Autodesk Inventor part; units mm, degrees
ref_plane "YZ Plane" through (0, 0, 0) normal (1, 0, 0) x (0, 1, 0)
ref_plane "XZ Plane" through (0, 0, 0) normal (0, 1, 0) x (-1, 0, 0)
ref_plane "XY Plane" through (0, 0, 0) normal (0, 0, 1) x (1, 0, 0)
sketch "Sketch1" plane through (0, 0, 0) normal (0, 0, 1) x (1, 0, 0)
  line L0 (17.5, -17.5) -> (0, -17.5)
  line L1 (-17.5, -17.5) -> (-17.5, 17.5)
  line L2 (-17.5, 17.5) -> (-7.5, 17.5) construction
  line L3 (17.5, 17.5) -> (17.5, 10)
  line L4 (17.5, -17.5) -> (-17.5, 17.5) construction
  line L5 (-17.5, -17.5) -> (17.5, 17.5) construction
  circle A0 centre (0, 0) radius 6.25
  line L6 (-17.5, -17.5) -> (-21.5, -17.5)
  line L7 (-21.5, -17.5) -> (-21.5, -7.5)
  line L8 (-21.5, -7.5) -> (-17.5, -7.5)
  line L9 (-17.5, -7.5) -> (-17.5, -17.5) construction
  line L10 (-17.5, 0) -> (-21.5, 0)
  line L11 (-21.5, 0) -> (-21.5, 10)
  line L12 (-21.5, 10) -> (-17.5, 10)
  line L13 (-17.5, 10) -> (-17.5, 0) construction
  line L14 (-17.5, 17.5) -> (-7.5, 17.5) construction
  line L15 (-7.5, 17.5) -> (-7.5, 21.5)
  line L16 (-7.5, 21.5) -> (-17.5, 21.5)
  line L17 (-17.5, 21.5) -> (-17.5, 17.5)
  line L18 (0, 17.5) -> (10, 17.5) construction
  line L19 (10, 17.5) -> (10, 21.5)
  line L20 (10, 21.5) -> (0, 21.5)
  line L21 (0, 21.5) -> (0, 17.5)
  line L22 (-17.5, 0) -> (17.5, 0) construction
  line L23 (0, -17.5) -> (0, 17.5) construction
  line L24 (-17.5, -17.5) -> (-7.5, -17.5)
  line L25 (-7.5, -17.5) -> (-7.5, -21.5)
  line L26 (-7.5, -21.5) -> (-17.5, -21.5)
  line L27 (-17.5, -21.5) -> (-17.5, -17.5)
  line L28 (0, -17.5) -> (10, -17.5) construction
  line L29 (10, -17.5) -> (10, -21.5)
  line L30 (10, -21.5) -> (0, -21.5)
  line L31 (0, -21.5) -> (0, -17.5)
  line L32 (17.5, -17.5) -> (21.5, -17.5)
  line L33 (21.5, -17.5) -> (21.5, -7.5)
  line L34 (21.5, -7.5) -> (17.5, -7.5)
  line L35 (17.5, -7.5) -> (17.5, -17.5) construction
  line L36 (17.5, 0) -> (21.5, 0)
  line L37 (21.5, 0) -> (21.5, 10)
  line L38 (21.5, 10) -> (17.5, 10)
  line L39 (17.5, 10) -> (17.5, 0) construction
  line L40 (-7.5, 17.5) -> (0, 17.5)
  line L41 (0, 17.5) -> (10, 17.5)
  line L42 (17.5, 10) -> (17.5, 0) construction
  line L43 (17.5, 0) -> (17.5, -7.5)
  line L44 (17.5, -7.5) -> (17.5, -17.5) construction
  line L45 (0, -17.5) -> (-17.5, -17.5)
  line L46 (10, 17.5) -> (17.5, 17.5)
  point P0 (0, 19.5)
  point P1 (-7.5, 19.5)
  point P2 (0, -19.5)
  point P3 (-7.5, -19.5)
  point P4 (-7.5, -17.5)
  point P5 (10, -17.5)
  dimension "d0" = 12.5
  dimension "d1" = 11.25
  dimension "d2" = 11.25
  dimension "d5" = 10
  dimension "d6" = 10
  dimension "d7" = 7.5
  dimension "d8" = 4
  dimension "d9" = 10
  dimension "d10" = 4
  dimension "d11" = 10
  dimension "d12" = 4
  dimension "d13" = 7.5
extrude "Extrusion1" add sketch "Sketch1" along normal blind 4
sketch "Sketch2" plane through (0, 0, 4) normal (0, 0, 1) x (1, 0, 0)
  line L0 (6.5, 17.5) -> (3.5, 17.5) construction
  line L1 (6.5, 21.5) -> (6.5, 17.5) construction
  line L2 (3.5, 21.5) -> (6.5, 21.5) construction
  line L3 (3.5, 21.5) -> (3.5, 17.5) construction
  line L4 (6.5, -21.5) -> (3.5, -21.5) construction
  line L5 (6.5, -17.5) -> (6.5, -21.5) construction
  line L6 (3.5, -17.5) -> (6.5, -17.5) construction
  line L7 (3.5, -17.5) -> (3.5, -21.5) construction
  line L8 (3.5, 17.5) -> (6.5, 21.5) construction
  line L9 (3.5, -17.5) -> (6.5, -21.5) construction
  circle A0 centre (5, 19.5) radius 1.5
  circle A1 centre (5, -19.5) radius 1.5
  point P0 (0, 0)
  dimension "d16" = 3
extrude "Extrusion2" cut sketch "Sketch2" against normal up to next
properties part number "FloorButtonHolder_Front_V1" material "MDF Medium Density Fiberboard"
Design review of the part built by this model. Coordinates are the model's own, in mm. A direction names the side the tool comes from. Give positions to 0.01 mm unless a question says otherwise; leave off trailing zeros. Order: outer loops, then holes, each group sorted by start corner. A loop starts at its lowest first (then second) coordinate and runs counter-clockwise, first axis right, second up. Notation, with made-up numbers: (50, 39) -> (64, 39) arc R18 cw to (64, 54) -> close; hole circle Ø1 at (-15.75, 47.5). An arc over 180 degrees is marked (long way). Write item = value, one per line. Start each with the question number.
(1) To check wall thickness, follow line 1 along Y through (x, z) = (19, 2.1); line 2 along Y through (x, z) = (5, 1.1); line 3 along X through (y, z) = (2, 0.65). State the ranges of each line that lie inside material, in increasing order.
(2) We need section C-C on x = -1.5. Write out the cut boundary in (y, z), plus the area to 3 significant figures.
(3) For faces 4 (the face through (-17.5, -4, 2)), 5 (the face through (-17.5, 16, 2)), 6 (the face through (-7.5, 19, 2)), 7 (the face through (10, 19, 2)), 8 (the face through (-17.5, -20, 2)), list the 3-axis set-ups (+Z, -Z, +X, -X, +Y, -Y) from which the entire face can be reached by the end or side of a thin tool; tool diameter is ignored.
(4) Mouldability with a two-part tool opening along X and no side actions: class faces 1 (the face through (-20, 10, 2)), 2 (the face through (0, 20, 2)), 3 (the face through (-21.5, 5, 2)) as +X half, -X half, draft (parallel to the pull), parting line (faces both ways), or undercut.
(5) We need section A-A on y = -19.5. Write out the cut boundary in (x, z), plus the area to 3 significant figures.
(6) We need section B-B on x = 5. Write out the cut boundary in (y, z), plus the area to 3 significant figures.
(7) For pin 1 (2 mm diameter, centred on x = 11.5, z = 3.5, fed in from -Y); pin 2 (1.2 mm diameter, centred on x = 19.5, z = 2, fed in from +Y); pin 3 (1.2 mm diameter, centred on x = 15.5, z = 1.5, fed in from +Y), all flat-tipped, find the tip position at first contact; note any pin that passes through.
(8) We need section D-D on y = -7. Write out the cut boundary in (x, z), plus the area to 3 significant figures.
Numbers:
q1.line_1 = -17.5 to -7.5, 0 to 10
q1.line_2 = -21.5 to -21, -18 to -3.75, 3.75 to 18, 21 to 21.5
q1.line_3 = -21.5 to -5.92, 5.92 to 21.5
q2.outline = (-17.5, 0) -> (-6.07, 0) -> (-6.07, 4) -> (-17.5, 4) -> close; (6.07, 0) -> (17.5, 0) -> (17.5, 4) -> (6.07, 4) -> close
q2.area = 91.5 mm^2
q3.face_4 = +Z, -Z, -X
q3.face_5 = +Z, -Z, -X, +Y
q3.face_6 = +Z, -Z, +Y
q3.face_7 = +Z, -Z, +X, +Y
q3.face_8 = +Z, -Z, -X, -Y
q4.face_1 = draft
q4.face_2 = undercut
q4.face_3 = -X half
q5.outline = (-17.5, 0) -> (-7.5, 0) -> (-7.5, 4) -> (-17.5, 4) -> close; (0, 0) -> (3.5, 0) -> (3.5, 4) -> (0, 4) -> close; (6.5, 0) -> (10, 0) -> (10, 4) -> (6.5, 4) -> close
q5.area = 68.0 mm^2
q6.outline = (-21.5, 0) -> (-21, 0) -> (-21, 4) -> (-21.5, 4) -> close; (-18, 0) -> (-3.75, 0) -> (-3.75, 4) -> (-18, 4) -> close; (3.75, 0) -> (18, 0) -> (18, 4) -> (3.75, 4) -> close; (21, 0) -> (21.5, 0) -> (21.5, 4) -> (21, 4) -> close
q6.area = 118 mm^2
q7.pin_1 = -17.5
q7.pin_2 = 10
q7.pin_3 = 17.5
q8.outline = (-17.5, 0) -> (17.5, 0) -> (17.5, 4) -> (-17.5, 4) -> close
q8.area = 140 mm^2
